from build123d import *

# Parameters (mm, degrees)
SALIENTE_EXTRUIR1_DEPTH      = 5
SALIENTE_EXTRUIR1_DEPTH_BACK = 20


with BuildPart() as part:
    # Croquis2 → Saliente-Extruir1 (new, two sides: drawn at the far end of the back side and taken through both)
    with BuildSketch(Plane.ZY.offset(192.754092983).offset(-SALIENTE_EXTRUIR1_DEPTH_BACK)):
        Polygon((334.847231333, 111.353262199), (334.847231333, -258.646737801), (156.847231333, -258.646737801), (-40.152768667, 86.353262199), (-40.152768667, 111.353262199), align=None)
    extrude(amount=SALIENTE_EXTRUIR1_DEPTH + SALIENTE_EXTRUIR1_DEPTH_BACK)


solid = part.part
Input: part model. Units: mm. Frame: model coordinates. Coordinates: 2 decimals unless noted, no trailing zeros. Loops run counter-clockwise (first coordinate to the right, second up) from the corner with the lowest first, then second, coordinate; pieces in that order, holes last. Notation, with made-up numbers: (76, 31) -> (88, 31) arc R30 ccw to (88, 63) -> close; hole circle Ø11 at (87.25, -39.75). An arc over 180 degrees is marked (long way). Write item = value, one per line. Start each with the question number.
Item 1: Material intervals for line 1 (Y direction, x = -176.25, z = 82); line 2 (Z direction, x = -183, y = 66); line 3 (Z direction, x = -184, y = -159.5), sorted ascending.
Item 2: Cut plane A-A, the plane x = -188. Return loops of the section in (y, z), plus the area to 3 significant figures.
Item 3: Cut plane B-B, the plane y = -236. Return loops of the section in (x, z).
Item 4: First-contact query: P1, Ø1, axis at x = -192.5, z = 129, coming from the -Y side; P2, Ø5, axis at x = -179.5, y = 35.5, coming from the -Z side; P3, Ø4, axis at x = -185.5, y = -103.5, coming from the -Z side. Flat tips, straight axial feed; report the tip coordinate or a pass-through.
Item 5: Cut plane C-C, the plane z = -9. Return loops of the section in (x, y).
Ans:
q1.line_1 = -127.57 to 111.35
q1.line_2 = -28.53 to 334.85
q1.line_3 = 100.23 to 334.85
q2.outline = (-258.65, 156.85) -> (86.35, -40.15) -> (111.35, -40.15) -> (111.35, 334.85) -> (-258.65, 334.85) -> close
q2.area = 105,000 mm²
q3.outline = (-197.75, 143.92) -> (-172.75, 143.92) -> (-172.75, 334.85) -> (-197.75, 334.85) -> close
q4.P1 = -210.75
q4.P2 = -12.54
q4.P3 = 67.11
q5.outline = (-197.75, 31.8) -> (-172.75, 31.8) -> (-172.75, 111.35) -> (-197.75, 111.35) -> close
